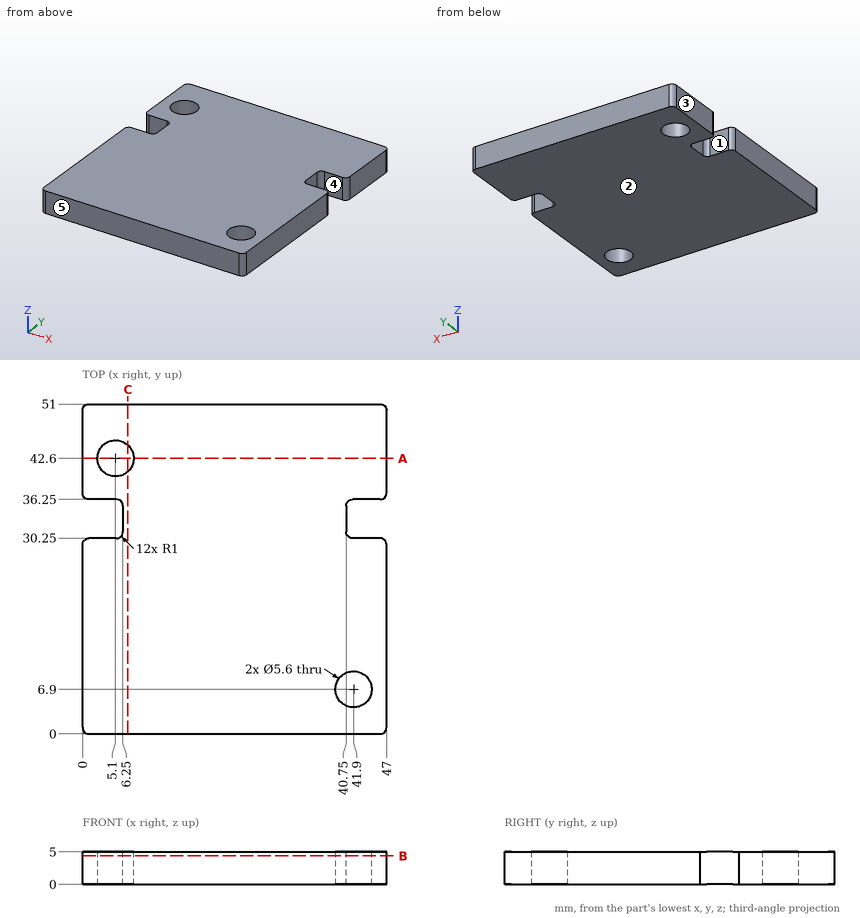
Can you work these out from the drawing? Everything is in mm from the part's minimum corner. A direction names the side the tool comes from. Coordinates: 2 decimals unless noted, no trailing zeros. Loops run counter-clockwise (first coordinate to the right, second up) from the corner with the lowest first, then second, coordinate; pieces in that order, holes last.
1) Imagine slicing it at B-B on z = 4.4. List the corners of the cut face in (x, y) for me.
2) Thinking about a two-plate mould opening in Y: for the marked faces 3, 4 and 5, which applies, pulls with the +Y half, pulls with the -Y half, needs draft (parallel to the pull), parting line crosses it, or undercut?
3) Imagine slicing it at C-C on x = 7. List the corners of the cut face in (y, z) for me, plus the area to 3 significant figures.
4) Imagine slicing it at A-A on y = 42.6. List the corners of the cut face in (x, z) for me.
5) For pin 1 (2 mm diameter, centred on y = 33.5, z = 3.5, fed in from +X), with a flat end and sliding along its axis, tell me the tip position at first contact or that it passes through.
6) Which directions (+Z, -Z, +X, -X, +Y, -Y) give clear straight access to the entire face, cutting with the end or side of a thin tool? Please do the marked faces 1 and 2.
7) I need wall thicknesses on probe 1 along Y at (x, z) = (41.9, 3.9); probe 2 along Y at (x, z) = (5.1, 3.55); probe 3 along X at (y, z) = (6.9, 1.85). Which ranges of each line are inside material? Lowest first, please.
Completed:
1. outline: (0, 1) arc R1 ccw to (1, 0) - (46, 0) arc R1 ccw to (47, 1) - (47, 29.25) arc R1 ccw to (46, 30.25) - (41.75, 30.25) arc R1 cw to (40.75, 31.25) - (40.75, 35.25) arc R1 cw to (41.75, 36.25) - (46, 36.25) arc R1 ccw to (47, 37.25) - (47, 50) arc R1 ccw to (46, 51) - (1, 51) arc R1 ccw to (0, 50) - (0, 37.25) arc R1 ccw to (1, 36.25) - (5.25, 36.25) arc R1 cw to (6.25, 35.25) - (6.25, 31.25) arc R1 cw to (5.25, 30.25) - (1, 30.25) arc R1 ccw to (0, 29.25) - close; hole circle Ø5.6 at (5.1, 42.6); hole circle Ø5.6 at (41.9, 6.9)
2. face 3: needs draft
2. face 4: undercut
2. face 5: pulls with the -Y half
3. outline: (0, 0) - (40.54, 0) - (40.54, 5) - (0, 5) - close; (44.66, 0) - (51, 0) - (51, 5) - (44.66, 5) - close
3. area: 234 mm2
4. outline: (0, 0) - (2.3, 0) - (2.3, 5) - (0, 5) - close; (7.9, 0) - (47, 0) - (47, 5) - (7.9, 5) - close
5. pin 1: stops at x = 40.75
6. face 1: +Z, -Z, -X
6. face 2: -Z, +X, -X, +Y, -Y
7. probe 1: y = 0 to 4.1, 9.7 to 30.25, 36.25 to 51
7. probe 2: y = 0 to 30.25, 36.25 to 39.8, 45.4 to 51
7. probe 3: x = 0 to 39.1, 44.7 to 47
